```python
from build123d import *

# Parameters (mm, degrees)
EXTRUDE_1_DEPTH     = 3
SKETCH_2_R          = 1.7
CUT_EXTRUDE_1_DEPTH = 117.764720699
SKETCH_3_W          = 15.4
SKETCH_3_H          = 2.2
CUT_EXTRUDE_2_DEPTH = 10
CUT_EXTRUDE_3_DEPTH = 10
FILLET_1_R          = 3
FILLET_2_R          = 3


with BuildPart() as part:
    # 草图1 → 凸台-拉伸1 (new body)
    with BuildSketch(Plane.XY):
        Polygon((0, 85), (0, 0), (80, 0), (80, 30), (61.422003178, 30), (20, 64.832139036), (20, 85), align=None)
        Polygon((20, 30), (20, 48.5), (42, 30), align=None, mode=Mode.SUBTRACT)
    extrude(amount=EXTRUDE_1_DEPTH)

    # 草图2 → 切除-拉伸1 (cut, through all)
    with BuildSketch(Plane.XY.offset(3)):
        with Locations((10, 75)):
            Circle(SKETCH_2_R)
        with Locations((10, 55)):
            Circle(SKETCH_2_R)
        with Locations((10, 35)):
            Circle(SKETCH_2_R)
        with Locations((30, 15)):
            Circle(SKETCH_2_R)
        with Locations((50, 15)):
            Circle(SKETCH_2_R)
        with Locations((70, 15)):
            Circle(SKETCH_2_R)
        with Locations((10, 15)):
            Circle(SKETCH_2_R)
    extrude(amount=-CUT_EXTRUDE_1_DEPTH, mode=Mode.SUBTRACT)

    # 草图3 → 切除-拉伸2 (cut)
    with BuildSketch(Plane.XY.offset(3)):
        with Locations((50, 26)):
            Rectangle(SKETCH_3_W, SKETCH_3_H)
        with Locations((50, 4)):
            Rectangle(SKETCH_3_W, SKETCH_3_H)
    extrude(amount=-CUT_EXTRUDE_2_DEPTH, mode=Mode.SUBTRACT)

    # 草图4 → 切除-拉伸3 (cut)
    with BuildSketch(Plane.XY.offset(3)):
        with BuildLine():
            Line((44.3, 27.1), (55.7, 27.1))
            ThreePointArc((55.7, 27.1), (56.7, 28.1), (57.7, 27.1))
            Line((57.7, 27.1), (57.7, 24.9))
            ThreePointArc((57.7, 24.9), (56.7, 23.9), (55.7, 24.9))
            Line((55.7, 24.9), (44.3, 24.9))
            ThreePointArc((44.3, 24.9), (43.3, 23.9), (42.3, 24.9))
            Line((42.3, 24.9), (42.3, 27.1))
            ThreePointArc((42.3, 27.1), (43.3, 28.1), (44.3, 27.1))
        make_face()
        with BuildLine():
            Line((42.3, 5.1), (42.3, 2.9))
            ThreePointArc((42.3, 2.9), (43.3, 1.9), (44.3, 2.9))
            Line((44.3, 2.9), (55.7, 2.9))
            ThreePointArc((55.7, 2.9), (56.7, 1.9), (57.7, 2.9))
            Line((57.7, 2.9), (57.7, 5.1))
            ThreePointArc((57.7, 5.1), (56.7, 6.1), (55.7, 5.1))
            Line((55.7, 5.1), (44.3, 5.1))
            ThreePointArc((44.3, 5.1), (43.3, 6.1), (42.3, 5.1))
        make_face()
    extrude(amount=-CUT_EXTRUDE_3_DEPTH, mode=Mode.SUBTRACT)

    # 圆角1
    fillet_1_edges = [part.edges().sort_by_distance(p)[0] for p in [
        (20, 85, 1.5),
        (20, 64.832139036, 1.5),
        (61.422003178, 30, 1.5),
        (80, 30, 1.5),
        (80, 0, 1.5),
        (0, 0, 1.5),
        (0, 85, 1.5),
    ]]
    fillet(fillet_1_edges, radius=FILLET_1_R)

    # 圆角2
    fillet_2_edges = [part.edges().sort_by_distance(p)[0] for p in [
        (20, 30, 1.5),
        (42, 30, 1.5),
        (20, 48.5, 1.5),
    ]]
    fillet(fillet_2_edges, radius=FILLET_2_R)


solid = part.part
```
Model file for the job. Use its own axes, mm. A direction names the side the tool comes from. Give positions to 0.01 mm unless a question says otherwise; leave off trailing zeros. Loops run counter-clockwise (first coordinate to the right, second up) from the corner with the lowest first, then second, coordinate; pieces in that order, holes last. Notation, with made-up numbers: M 50.5,-36.75 L 60.5,-36.75 A25 ccw 60.5,-8.75 Z; hole C -30.5,85 d9. An arc over 180 degrees is marked long. Use one line per item in the form item = value.
Item 1: Slice it at C-C on x = 70. List the corners of the cut face in (y, z), and give its area (3 significant figures).
Filled in:
outline = M 0,0 L 13.3,0 L 13.3,3 L 0,3 Z; M 16.7,0 L 30,0 L 30,3 L 16.7,3 Z
area = 79.8 mm^2
Item 2: Slice it at B-B on x = 10. List the corners of the cut face in (y, z), and give its area (3 significant figures).
Filled in:
outline = M 0,0 L 13.3,0 L 13.3,3 L 0,3 Z; M 16.7,0 L 33.3,0 L 33.3,3 L 16.7,3 Z; M 36.7,0 L 53.3,0 L 53.3,3 L 36.7,3 Z; M 56.7,0 L 73.3,0 L 73.3,3 L 56.7,3 Z; M 76.7,0 L 85,0 L 85,3 L 76.7,3 Z
area = 214 mm^2
Item 3: Slice it at D-D on x = 30.5. List the corners of the cut face in (y, z).
Filled in:
outline = M 0,0 L 13.38,0 L 13.38,3 L 0,3 Z; M 16.62,0 L 30,0 L 30,3 L 16.62,3 Z; M 39.67,0 L 56,0 L 56,3 L 39.67,3 Z
Item 4: Which spindle directions (+Z, -Z, +X, -X, +Y, -Y) get a long thin tool onto all of the face, cutting with end or side? Do faces 4 (the cylindrical face through (36.57, 31.92, 1.52)), 5 (the cylindrical face through (19.1, 84.14, 1.52)). Say none if no direction does.
Filled in:
face_4 = +Z, -Z
face_5 = +Z, -Z, +X, +Y
Item 5: Two-plate mould, pull along Y, no slides. Class faces 1 (the flat face through (31, 24, 3)), 2 (the cylindrical face through (56.7, 23.9, 1.5)), 3 (the cylindrical face through (79.14, 29.1, 1.52)): released by +Y, released by -Y, zero draft, split by the parting line, or undercut.
Filled in:
face_1 = zero draft
face_2 = undercut
face_3 = released by +Y
Item 6: Drill centre lines: L1, parallel to Y at x = 10, z = 2.2; L2, parallel to Y at x = 44, z = 2.1; L3, parallel to X at y = 26, z = 1.9. Where is each one in solid material? Low to high.
Filled in:
L1 = 0 to 13.3, 16.7 to 33.3, 36.7 to 53.3, 56.7 to 73.3, 76.7 to 85
L2 = 0 to 2.19, 5.81 to 24.19, 27.81 to 44.65
L3 = 0 to 42.3, 57.7 to 80
Item 7: Flat gauge pins, fed straight in: pin 1 Ø1.5 at (x, z) = (69.5, 1.5) entering from +Y; pin 2 Ø1.5 at (x, z) = (52, 1) entering from +Y; pin 3 Ø1.5 at (x, z) = (30, 2) entering from +Y. Where does each tip first touch, or does it go through?
Filled in:
pin_1 = 30
pin_2 = 38.55
pin_3 = 57.05
Item 8: Slice it at A-A on y = 75. List the corners of the cut face in (x, z).
Filled in:
outline = M 0,0 L 8.3,0 L 8.3,3 L 0,3 Z; M 11.7,0 L 20,0 L 20,3 L 11.7,3 Z
